Here's how the part is built. I have some questions about the finished solid (model axes, mm). A direction names the side the tool comes from. Round coordinates to 2 decimals unless told otherwise and drop trailing zeros. Loops run counter-clockwise (first coordinate to the right, second up) from the corner with the lowest first, then second, coordinate; pieces in that order, holes last. Notation, with made-up numbers: (12.25, 59.25) -> (33.25, 59.25) arc R24 ccw to (33.25, 88.25) -> close; hole circle Ø3 at (-21, 27.25). An arc over 180 degrees is marked (long way). Use CSV: the item, a comma, the result in double quotes. Start each with the question number.
from build123d import *

# Parameters (mm, degrees)
SKETCH_1_W          = 100
SKETCH_1_H          = 118
EXTRUDE_1_DEPTH     = 3
SKETCH_3_R          = 1.5
CUT_EXTRUDE_2_DEPTH = 3
SKETCH_4_R          = 2.5
CUT_EXTRUDE_3_DEPTH = 3
SKETCH_5_R          = 1.5
CUT_EXTRUDE_4_DEPTH = 3
CUT_EXTRUDE_6_DEPTH = 3
SKETCH_9_R          = 1.5
CUT_EXTRUDE_8_DEPTH = 10
FILLET_3_R          = 5


with BuildPart() as part:
    # Sketch 1 → Extrude 1 (new body)
    with BuildSketch(Plane(origin=(0, 0, 0), x_dir=(1, 0, 0), z_dir=(0, 1, 0))):
        Rectangle(SKETCH_1_W, SKETCH_1_H)
    extrude(amount=EXTRUDE_1_DEPTH)

    # Sketch 3 → Cut-Extrude 2 (cut)
    with BuildSketch(Plane(origin=(0, 3, 0), x_dir=(1, 0, 0), z_dir=(0, 1, 0))):
        with Locations(Location((3.5, -1.5, 0), (0, 0, 270))):
            Circle(SKETCH_3_R)
        with Locations(Location((45.5, -1.5, 0), (0, 0, 90))):
            Circle(SKETCH_3_R)
        with Locations(Location((45.5, -26.5, 0), (0, 0, 270))):
            Circle(SKETCH_3_R)
        with Locations(Location((3.5, -26.5, 0), (0, 0, 90))):
            Circle(SKETCH_3_R)
    extrude(amount=-CUT_EXTRUDE_2_DEPTH, mode=Mode.SUBTRACT)

    # Sketch 4 → Cut-Extrude 3 (cut)
    with BuildSketch(Plane(origin=(0, 3, 0), x_dir=(1, 0, 0), z_dir=(0, 1, 0))):
        with Locations(Location((37.5, 52, 0), (0, 0, 270))):
            Circle(SKETCH_4_R)
        with Locations(Location((19.7, 52, 0), (0, 0, 90))):
            Circle(SKETCH_4_R)
        with Locations(Location((-19.7, 52, 0), (0, 0, 270))):
            Circle(SKETCH_4_R)
        with Locations(Location((-37.5, 52, 0), (0, 0, 90))):
            Circle(SKETCH_4_R)
    extrude(amount=-CUT_EXTRUDE_3_DEPTH, mode=Mode.SUBTRACT)

    # Sketch 5 → Cut-Extrude 4 (cut)
    with BuildSketch(Plane(origin=(0, 3, 0), x_dir=(1, 0, 0), z_dir=(0, 1, 0))):
        with Locations(Location((22, -54, 0), (0, 0, 270))):
            Circle(SKETCH_5_R)
        with Locations(Location((14, -54, 0), (0, 0, 90))):
            Circle(SKETCH_5_R)
    extrude(amount=-CUT_EXTRUDE_4_DEPTH, mode=Mode.SUBTRACT)

    # Sketch 7 → Cut-Extrude 6 (cut)
    with BuildSketch(Plane(origin=(0, 3, 0), x_dir=(1, 0, 0), z_dir=(0, 1, 0))):
        Polygon((-24.285714286, -49), (-50, 11), (-50, -59), (-20, -59), align=None)
        Polygon((-4.285714286, -49), (-24.285714286, -49), (-20, -59), (0, -59), align=None)
    extrude(amount=-CUT_EXTRUDE_6_DEPTH, mode=Mode.SUBTRACT)

    # Sketch 9 → Cut-Extrude 8 (cut)
    with BuildSketch(Plane(origin=(0, 3, 0), x_dir=(1, 0, 0), z_dir=(0, 1, 0))):
        with Locations(Location((-22, -41, 0), (0, 0, 270))):
            Circle(SKETCH_9_R)
        with Locations(Location((-10, -41, 0), (0, 0, 270))):
            Circle(SKETCH_9_R)
    extrude(amount=-CUT_EXTRUDE_8_DEPTH, mode=Mode.SUBTRACT)

    # Fillet 3
    fillet_3_edges = [part.edges().sort_by_distance(p)[0] for p in [
        (0, 1.5, 59),
        (-50, 1.5, -11),
        (-24.285714286, 1.5, 49),
        (-4.285714286, 1.5, 49),
        (50, 1.5, 59),
        (-50, 1.5, -59),
        (50, 1.5, -59),
    ]]
    fillet(fillet_3_edges, radius=FILLET_3_R)


solid = part.part
Q1. For faces 1 (the flat face through (-14, 2, 49)), 2 (the flat face through (-1, 3, -1)), which set-ups out of +Z, -Z, +X, -X, +Y, -Y let a thin tool reach every point of the face, with its end or its side?
Q2. I want a section at B-B, the plane z = -52. List the corners of the cut face in (x, y) for me, then the cut area to 3 significant figures.
Q3. If we mould it in two halves opening along X, with no side actions, what happens to faces 3 (the flat face through (-50, 1, -33)), 4 (the flat face through (-1, 1, -59)), 5 (the cylindrical face through (-10.9, 1.5, 39.8)), 6 (the cylindrical face through (48, 2, -58))? For each: pulls with the +X half, pulls with the -X half, needs draft (parallel to the pull), parting line crosses it, or undercut.
Q4. I want a section at A-A, the plane x = -10. List the corners of the cut face in (y, z) for me.
Q5. I want a section at C-C, the plane y = 2.35. Count the separate pieces of the cut face and the enclosed holes in it, then the cut area to 3 significant figures.
Q6. I need wall thicknesses on line 1 along X through (y, z) = (1.55, -52); line 2 along Z through (x, y) = (14, 0.5); line 3 along Z through (x, y) = (19.7, 1.15). Which ranges of each line are inside material? Lowest first, please.
Q7. Will this pin go through, and if not, where does the flat tip stop? pin 1 Ø1.5 at (x, y) = (-16, 1.5) entering from +Z.
Q8. I want a section at D-D, the plane z = 26.5. List the corners of the cut face in (x, y) for me, then the cut area to 3 significant figures.
Values found:
1,face 1,"+Z, -X, +Y, -Y"
1,face 2,"+Z, -Z, +X, -X, +Y"
2,outline,"(-50, 0) -> (-40, 0) -> (-40, 3) -> (-50, 3) -> close; (-35, 0) -> (-22.2, 0) -> (-22.2, 3) -> (-35, 3) -> close; (-17.2, 0) -> (17.2, 0) -> (17.2, 3) -> (-17.2, 3) -> close; (22.2, 0) -> (35, 0) -> (35, 3) -> (22.2, 3) -> close; (40, 0) -> (50, 0) -> (50, 3) -> (40, 3) -> close"
2,area,"240 mm2"
3,face 3,"pulls with the -X half"
3,face 4,"needs draft"
3,face 5,"undercut"
3,face 6,"pulls with the +X half"
4,outline,"(0, -59) -> (3, -59) -> (3, 39.5) -> (0, 39.5) -> close; (0, 42.5) -> (3, 42.5) -> (3, 49) -> (0, 49) -> close"
5,separate pieces,"1"
5,enclosed holes,"12"
5,area,"10,400 mm2"
6,line 1,"-50 to -40, -35 to -22.2, -17.2 to 17.2, 22.2 to 35, 40 to 50"
6,line 2,"-59 to 52.5, 55.5 to 59"
6,line 3,"-59 to -54.5, -49.5 to 59"
7,pin 1,"z = 49"
8,outline,"(-33.93, 0) -> (2, 0) -> (2, 3) -> (-33.93, 3) -> close; (5, 0) -> (44, 0) -> (44, 3) -> (5, 3) -> close; (47, 0) -> (50, 0) -> (50, 3) -> (47, 3) -> close"
8,area,"234 mm2"
